from build123d import *

# Parameters (mm, degrees)
CYLINDER_R           = 1.3
CYLINDER_DEPTH       = 50
CYLINDER_PITCH_ANGLE = -90
SKETCH_R             = 12.158698
PAD_DEPTH            = 60
SKETCH001_R          = 11.129855
POCKET_DEPTH         = 59
PAD001_DEPTH         = 60
SKETCH003_W          = 5.624389
SKETCH003_H          = 8.223541
POCKET001_DEPTH      = 0.5
PAD002_DEPTH         = 36


with BuildPart() as cylinder:
    # Cylinder → Cylinder (new body)
    with BuildSketch(Plane.XY):
        Circle(CYLINDER_R)
    extrude(amount=CYLINDER_DEPTH)


with BuildPart() as cylinder_1:
    # Cylinder pitch: moved
    add(cylinder.part.rotate(Axis((0, 0, 0), (0, 1, 0)), CYLINDER_PITCH_ANGLE))


with BuildPart() as cylinder_2:
    # Cylinder placement: moved
    add(cylinder_1.part.moved(Location((25, 0, 38.5))))


with BuildPart() as cut:
    # Sketch → Pad (new body)
    with BuildSketch(Plane.XY):
        Circle(SKETCH_R)
    extrude(amount=PAD_DEPTH)

    # Sketch001 (on Face3 of Pad) → Pocket (cut)
    with BuildSketch(Plane.XY.offset(60)):
        Circle(SKETCH001_R)
    extrude(amount=-POCKET_DEPTH, mode=Mode.SUBTRACT)

    # Sketch002 → Pad001 (join)
    with BuildSketch(Plane.XY):
        with BuildLine():
            Line((2.805862, 9.68487), (2.805862, -9.68487))
            ThreePointArc((2.805862, -9.68487), (10.083133, 0), (2.805862, 9.68487))
        make_face()
        with BuildLine():
            Line((-2.818532, -9.684849), (-2.818532, 9.684849))
            ThreePointArc((-2.818532, 9.684849), (-10.086646, 0), (-2.818532, -9.684849))
        make_face()
    extrude(amount=PAD001_DEPTH)

    # Sketch003 (on Face7 of Pad001) → Pocket001 (cut)
    with BuildSketch(Plane.XY.offset(1)):
        with Locations((-0.021016, 0.484692)):
            Rectangle(SKETCH003_W, SKETCH003_H)
    extrude(amount=-POCKET001_DEPTH, mode=Mode.SUBTRACT)

    # Sketch004 (on Face7 of Pocket001) → Pad002 (join)
    with BuildSketch(Plane.XY.offset(1)):
        with BuildLine():
            ThreePointArc((-3.168719, 10.816817), (-11.271375, -0.02054), (-3.129274, -10.828294))
            Line((-2.766472, -9.520992), (-3.129274, -10.828294))
            ThreePointArc((-2.764641, 9.521524), (-9.91477, 0.000953), (-2.766472, -9.520992))
            Line((-3.168719, 10.816817), (-2.764641, 9.521524))
        make_face()
        with BuildLine():
            ThreePointArc((10.639772, -3.318351), (11.124371, 0.350816), (10.384091, 3.977054))
            Line((9.22397, 3.5596), (10.384091, 3.977054))
            ThreePointArc((9.444413, -2.924966), (9.881272, 0.335915), (9.22397, 3.5596))
            Line((9.444413, -2.924966), (10.639772, -3.318351))
        make_face()
    extrude(amount=PAD002_DEPTH)

    # Cut: cut Cylinder
    add(cylinder_2.part, mode=Mode.SUBTRACT)


solid = cut.part
Can you work these out from the model? Positions are in its coordinate system, mm. A direction names the side the tool comes from. Round coordinates to 2 decimals unless told otherwise and drop trailing zeros. Loops run counter-clockwise (first coordinate to the right, second up) from the corner with the lowest first, then second, coordinate; pieces in that order, holes last. Notation, with made-up numbers: (40, 45) - (90, 45) arc R26 ccw to (90, 66) - close; hole circle Ø9 at (34.25, 11). An arc over 180 degrees is marked (long way). Answer in a Markdown table with one row per item. Add a question column.
Q1. I need wall thicknesses on L1, parallel to Y at x = 0, z = 33.5; L2, parallel to Z at x = 11.7, y = 0; L3, parallel to Y at x = 3.75, z = 12. Which ranges of each line are inside material? Lowest first, please.
Q2. I want a section at A-A on z = 17. List the corners of the cut face in (x, y) for me.
Q3. I want a section at C-C on x = -9.25. List the corners of the cut face in (y, z) for me.
Q4. For pin 1 Ø8 at (y, z) = (-5, 34.5) entering from +X; pin 2 Ø2 at (x, z) = (-5.5, 29) entering from +Y; pin 3 Ø10 at (y, z) = (-8, 20.5) entering from -X, each with a flat end and sliding along its axis, tell me the tip position at first contact or that it passes through.
Q5. I want a section at B-B on z = 38.5. List the corners of the cut face in (x, y) for me, and give its area (3 significant figures).
Q6. Which directions (+Z, -Z, +X, -X, +Y, -Y) give clear straight access to the entire face, cutting with the end or side of a thin tool? Please do faces 1 (the flat face through (-10.4, -0.7, 37)), 2 (the flat face through (11, -4, 60)).
Q7. I want a section at D-D on x = 0. List the corners of the cut face in (y, z) for me, and give its area (3 significant figures).
Q8. We'd pull the mould along Y, two halves only. Please class faces 3 (the flat face through (0, 1, 0.5)), 4 (the flat face through (6, 0, 60)): pulls with the +Y half, pulls with the -Y half, needs draft (parallel to the pull), parting line crosses it, or undercut.
A:
| question | item | result |
|---|---|---|
| 1 | L1 | -12.16 to -11.13, 11.13 to 12.16 |
| 1 | L2 | 0 to 37.2, 39.8 to 60 |
| 1 | L3 | -11.57 to -10.48, -9.36 to 9.36, 10.48 to 11.57 |
| 2 | outline | circle Ø24.32 at (0, 0); hole (-3.13, 10.68) - (-2.76, 9.52) arc R9.91 ccw to (-2.82, 9.51) - (-2.82, -9.51) arc R9.91 ccw to (-2.77, -9.52) - (-3.09, -10.69) arc R11.13 ccw to (10.63, -3.31) - (9.63, -2.99) arc R10.08 cw to (2.81, -9.68) - (2.81, 9.68) arc R10.08 cw to (9.41, 3.63) - (10.38, 3.98) arc R11.18 cw to (11.12, 0.36) arc R11.13 ccw to start |
| 3 | outline | (-7.89, 0) - (7.89, 0) - (7.89, 60) - (6.19, 60) - (6.19, 37) - (4.02, 37) - (4.02, 60) - (-4.02, 60) - (-4.02, 37) - (-6.19, 37) - (-6.19, 60) - (-7.89, 60) - close; hole circle Ø2.6 at (0, 38.5) |
| 4 | pin 1 | x = 12.12 |
| 4 | pin 2 | y = 11.3 |
| 4 | pin 3 | x = -11.78 |
| 5 | outline | (-12.09, -1.3) arc R12.16 ccw to (12.09, -1.3) - (11.05, -1.3) arc R11.13 cw to (-11.05, -1.3) - close; (-12.09, 1.3) - (-11.05, 1.3) arc R11.13 cw to (11.05, 1.3) - (12.09, 1.3) arc R12.16 ccw to start; (-10, -1.3) arc R10.09 ccw to (-2.82, -9.68) - (-2.82, -1.3) - close; (-10, 1.3) - (-2.82, 1.3) - (-2.82, 9.68) arc R10.09 ccw to start; (2.81, -9.68) arc R10.08 ccw to (10, -1.3) - (2.81, -1.3) - close; (2.81, 1.3) - (10, 1.3) arc R10.08 ccw to (2.81, 9.68) - close |
| 5 | area | 240 mm^2 |
| 6 | face 1 | +Z |
| 6 | face 2 | +Z, +X, -X, +Y, -Y |
| 7 | outline | (-12.16, 0) - (12.16, 0) - (12.16, 60) - (11.13, 60) - (11.13, 1) - (4.6, 1) - (4.6, 0.5) - (-3.63, 0.5) - (-3.63, 1) - (-11.13, 1) - (-11.13, 60) - (-12.16, 60) - close |
| 7 | area | 142 mm^2 |
| 8 | face 3 | undercut |
| 8 | face 4 | needs draft |
